```python
from build123d import *

# Parameters (mm, degrees)
BODY001_PLACEMENT_ANGLE = 45
PAD_DEPTH               = 80
SKETCH001_W             = 2.5
SKETCH001_H             = 6
POCKET_DEPTH            = 28.674996
FILLET_R                = 2
FILLET001_R             = 1


with BuildPart() as body001:
    # Sketch002 → Revolution (revolve)
    with BuildSketch(Plane.YZ):
        Polygon((0, 0), (0, 6.15), (28, 6.15), (28, 10.25), (56.26033, 10.25), (56.26033, 0), align=None)
    revolve(axis=Axis((0, 0, 0), (0, 1, 0)))


with BuildPart() as body001_1:
    # Body001 placement: moved
    add(body001.part.moved(Location((0, 9, 31))).rotate(Axis((0, 9, 31), (1, 0, 0)), BODY001_PLACEMENT_ANGLE))


with BuildPart() as fillet001:
    # Sketch → Pad (new body)
    with BuildSketch(Plane.XY):
        with BuildLine():
            ThreePointArc((0, 3.83), (-4, 2.758203), (-6.928203, -0.17))
            Line((-6.928203, -0.17), (-11.835681, -8.67))
            ThreePointArc((-11.835681, -8.67), (-12.505553, -11.17), (-11.835681, -13.67))
            ThreePointArc((-14.551626, -14.912315), (-12.510772, -15.784071), (-11.835681, -13.67))
            ThreePointArc((-13.807272, 0.232263), (-15.649568, -7.26777), (-14.551626, -14.912315))
            ThreePointArc((-13.807272, 0.232263), (-13.204197, 2.02521), (-13, 3.905811))
            Line((-13, 3.905811), (-13, 33.83))
            ThreePointArc((-11, 35.83), (-12.414214, 35.244214), (-13, 33.83))
            Line((-11, 35.83), (0, 35.83))
            Line((0, 35.83), (0, 3.83))
        make_face()
    pad = extrude(amount=PAD_DEPTH)

    # Mirrored: Pad across Sketch V_Axis
    add(pad.mirror(Plane(origin=(0, 0, 0), x_dir=(0, 0, 1), z_dir=(1, 0, 0))))

    # Sketch001 (on Face20 of Mirrored) → Pocket (cut, through all)
    with BuildSketch(Plane.YZ.offset(13)):
        with Locations((7.516462, 70.611825)):
            Rectangle(SKETCH001_W, SKETCH001_H)
        with Locations((7.516462, 9.388175)):
            Rectangle(SKETCH001_W, SKETCH001_H)
        Polygon((9.062247, -7.596541), (45.172724, 43.974565), (45.172724, -7.596541), align=None)
        Polygon((20.480662, 90.329349), (40.583266, 70.226745), (40.583266, 96.418373), align=None)
    extrude(amount=-POCKET_DEPTH, mode=Mode.SUBTRACT)

    # Cut: cut Body001
    add(body001_1.part, mode=Mode.SUBTRACT)

    # Fillet
    fillet_edges = [fillet001.edges().sort_by_distance(p)[0] for p in [
        (-13, 24.105701, 13.887738),
        (13, 24.105701, 13.887738),
    ]]
    fillet(fillet_edges, radius=FILLET_R)

    # Fillet001
    fillet001_edges = [fillet001.edges().sort_by_distance(p)[0] for p in [
        (-13, 32.320005, 78.490005),
        (-6.5, 30.810011, 80),
        (-12.526592, 35.122098, 75.687913),
        (13, 32.320005, 78.490005),
        (12.526592, 35.122098, 75.687913),
        (5.5, 35.83, 74.980011),
        (-5.5, 35.83, 74.980011),
        (6.5, 30.810011, 80),
    ]]
    fillet(fillet001_edges, radius=FILLET001_R)


solid = fillet001.part
```
Verification items for the finished model (mm, model axes). A direction names the side the tool comes from. Give positions to 0.01 mm unless a question says otherwise; leave off trailing zeros. Loops run counter-clockwise (first coordinate to the right, second up) from the corner with the lowest first, then second, coordinate; pieces in that order, holes last. Notation, with made-up numbers: M 44,-11 L 69,-11 A11 ccw 69,-4 Z; hole C -36.75,70 d4. An arc over 180 degrees is marked long. One line per question, with ' | ' between items.
Item 1: Section check B-B, the plane x = -1.5. Record the cut outline in (y, z), plus the area to 3 significant figures.
Completed:
outline: M 3.69,0 L 14.38,0 L 35.47,30.12 A2 ccw 35.83,31.26 L 35.83,43.77 L 33.02,46.58 L 13.22,26.78 L 4.78,35.22 L 24.58,55.02 L 21.63,57.97 L 35.83,72.17 L 35.83,74.57 A1 ccw 35.54,75.27 L 31.1,79.71 A1 ccw 30.4,80 L 3.69,80 Z; hole M 6.27,6.39 L 8.77,6.39 L 8.77,12.39 L 6.27,12.39 Z; hole M 6.27,67.61 L 8.77,67.61 L 8.77,73.61 L 6.27,73.61 Z | area: 1,660 mm^2
Item 2: Tool access check on faces 1 (the face through (-13, 19, 48)), 2 (the face through (0, 13, 80)), 3 (the face through (4.7, 31.8, 47.8)), 4 (the face through (0, 7, 67.612)). Record the directions out of +Z, -Z, +X, -X, +Y, -Y that give a thin tool (end or side, any length) a straight path to the whole face; none if there is none.
Completed:
face 1: +Z, -Z, -X, +Y | face 2: +Z, +X, -X, +Y, -Y | face 3: none | face 4: +X, -X
Item 3: Section check C-C, the plane y = 7.5. State how many separate pieces and enclosed holes the cut face has, plus the area to 3 significant figures.
Completed:
separate pieces: 3 | enclosed holes: 1 | area: 1,720 mm^2
Item 4: Depth check by flat-ended pin: P1, Ø5, axis at x = 6, z = 69.5, coming from the -Y side; P2, Ø4, axis at x = -2.5, z = 15.5, coming from the -Y side; P3, Ø10, axis at x = -0.5, y = -3.5, coming from the -Z side; P4, Ø1, axis at y = 0, z = 69.5, coming from the -X side. Enter the tip coordinate at first touch or a pass-through.
Completed:
P1: stops at y = -2.89 | P2: stops at y = 2.44 | P3: passes through | P4: stops at x = -14.13
Item 5: Thickness scan on line 1 (Z direction, x = -9, y = 8.5); line 2 (Y direction, x = -12, z = 70); line 3 (Y direction, x = -12, z = 8.5). Record the ranges inside material, lowest first. Write a range as [from, to].
Completed:
line 1: z = [0, 6.39], [12.39, 67.61], [73.61, 80] | line 2: y = [-15.4, -13.36], [-8.98, 6.27], [8.77, 35.56] | line 3: y = [-15.4, -13.36], [-8.98, 6.27], [8.77, 20.01]
Item 6: Section check A-A, the plane y = -7. Record the cut outline in (x, z).
Completed:
outline: M -15.63,0 L -10.87,0 L -10.87,80 L -15.63,80 Z; M 10.87,0 L 15.63,0 L 15.63,80 L 10.87,80 Z
Item 7: Draft check along Y on faces 5 (the face through (13, 19, 48)), 6 (the face through (12.4, 35.26, 53.06)), 7 (the face through (-15.644, -7.159, 39.44)), 8 (the face through (0, 6.266, 9)). Enter one of: +Y half, -Y half, draft (parallel to the pull), parting line (faces both ways), or undercut.
Completed:
face 5: draft | face 6: +Y half | face 7: parting line | face 8: undercut
Item 8: Section check D-D, the plane x = 8.5. Record the cut outline in (y, z), plus the area to 3 significant figures.
Completed:
outline: M -2.89,0 L 14.38,0 L 35.47,30.12 A2 ccw 35.83,31.26 L 35.83,49.73 L 32.85,46.75 L 24.75,54.85 L 35.83,65.93 L 35.83,74.57 A1 ccw 35.54,75.27 L 31.1,79.71 A1 ccw 30.4,80 L -2.89,80 Z; hole M 6.27,6.39 L 8.77,6.39 L 8.77,12.39 L 6.27,12.39 Z; hole M 6.27,67.61 L 8.77,67.61 L 8.77,73.61 L 6.27,73.61 Z | area: 2,610 mm^2
